Here's how the part is built. I have some questions about the finished solid (model axes, mm). Round coordinates to 2 decimals unless told otherwise and drop trailing zeros. Write each loop counter-clockwise with the first axis right and the second up, starting at its lowest first coordinate (ties: lowest second). Pieces come first, ordered by that corner, then holes. Notation, with made-up numbers: (-18.75, -8) - (39.25, -8) arc R26 cw to (39.25, 18) - close; hole circle Ø2 at (86.5, 60). An arc over 180 degrees is marked (long way). Write item = value, one per line. Start each with the question number.
Item 1: If we section it at C-C (x = 10): Please give me the cut outline in (y, z).
Item 2: If we section it at D-D (y = 0.55): Please give me the cut outline in (x, z).
Item 3: For P1, Ø4.5, axis at x = 35, z = -45, coming from the -Y side, with a flat end and sliding along its axis, tell me the tip position at first contact or that it passes through.
Item 4: If we section it at B-B (z = -10): Please give me the cut outline in (x, y).
Item 5: If we section it at A-A (z = -45): Please give me the cut outline in (x, y).
Item 6: If I drill on line 1 along X through (y, z) = (2.2, -45); line 2 along Z through (x, y) = (36, 2.5); line 3 along X through (y, z) = (0.65, -46), over which ranges is the centre line in solid material (lowest first)? Write a range as [from, to].
```python
from build123d import *

# Parameters (mm, degrees)
SKETCH1_W           = 50
SKETCH1_H           = 50
BOSS_EXTRUDE1_DEPTH = 3
SKETCH2_R           = 2.0066
CUT_EXTRUDE1_DEPTH  = 4
CUT_EXTRUDE2_REACH  = 5
SKETCH3_R           = 1.45


with BuildPart() as part:
    # Sketch1 → Boss-Extrude1 (new body)
    with BuildSketch(Plane(origin=(0, 0, 0), x_dir=(1, 0, 0), z_dir=(0, 1, 0))):
        with Locations((25, 25)):
            Rectangle(SKETCH1_W, SKETCH1_H)
    extrude(amount=BOSS_EXTRUDE1_DEPTH)

    # Sketch2 → Cut-Extrude1 (cut, through all)
    with BuildSketch(Plane(origin=(0, 3, 0), x_dir=(1, 0, 0), z_dir=(0, 1, 0))):
        with Locations((10, 45)):
            Circle(SKETCH2_R)
        with Locations((35, 45)):
            Circle(SKETCH2_R)
        with Locations((10, 10)):
            Circle(SKETCH2_R)
    extrude(amount=-CUT_EXTRUDE1_DEPTH, mode=Mode.SUBTRACT)

    # Sketch3 → Cut-Extrude2 (cut, up to next)
    with BuildSketch(Plane(origin=(0, 3, 0), x_dir=(1, 0, 0), z_dir=(0, 1, 0)), mode=Mode.PRIVATE) as cut_extrude2_sk1:
        with Locations((47.301711452, 25.073921106)):
            Circle(SKETCH3_R)
    cut_extrude2_tool1 = extrude(cut_extrude2_sk1.sketch, amount=-CUT_EXTRUDE2_REACH, mode=Mode.PRIVATE) & part.part
    add(cut_extrude2_tool1.solids().sort_by_distance((47.301711, 3, -25.073921))[0], mode=Mode.SUBTRACT)
    # Sketch3 → Cut-Extrude2 (cut, up to next)
    with BuildSketch(Plane(origin=(0, 3, 0), x_dir=(1, 0, 0), z_dir=(0, 1, 0)), mode=Mode.PRIVATE) as cut_extrude2_sk2:
        with Locations((37.001711452, 2.873921106)):
            Circle(SKETCH3_R)
    cut_extrude2_tool2 = extrude(cut_extrude2_sk2.sketch, amount=-CUT_EXTRUDE2_REACH, mode=Mode.PRIVATE) & part.part
    add(cut_extrude2_tool2.solids().sort_by_distance((37.001711, 3, -2.873921))[0], mode=Mode.SUBTRACT)


solid = part.part
```
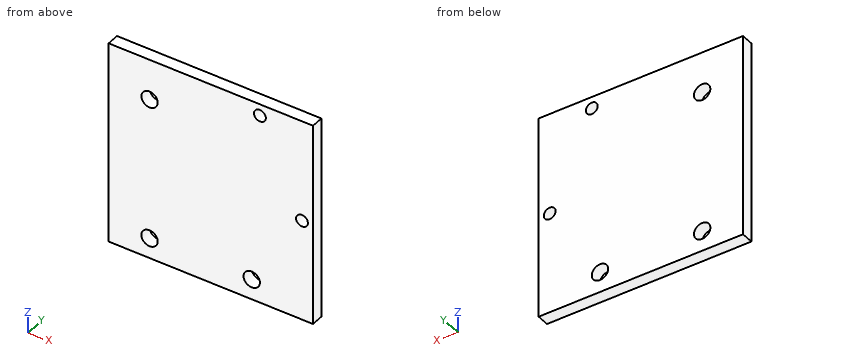
Reply:
q1.outline = (0, -50) - (3, -50) - (3, -47.01) - (0, -47.01) - close; (0, -42.99) - (3, -42.99) - (3, -12.01) - (0, -12.01) - close; (0, -7.99) - (3, -7.99) - (3, 0) - (0, 0) - close
q2.outline = (0, -50) - (50, -50) - (50, 0) - (0, 0) - close; hole circle Ø4.01 at (10, -45); hole circle Ø4.01 at (10, -10); hole circle Ø4.01 at (35, -45); hole circle Ø2.9 at (37, -2.87); hole circle Ø2.9 at (47.3, -25.07)
q3.P1 = 0
q4.outline = (0, 0) - (7.99, 0) - (7.99, 3) - (0, 3) - close; (12.01, 0) - (50, 0) - (50, 3) - (12.01, 3) - close
q5.outline = (0, 0) - (7.99, 0) - (7.99, 3) - (0, 3) - close; (12.01, 0) - (32.99, 0) - (32.99, 3) - (12.01, 3) - close; (37.01, 0) - (50, 0) - (50, 3) - (37.01, 3) - close
q6.line_1 = [0, 7.99], [12.01, 32.99], [37.01, 50]
q6.line_2 = [-50, -46.74], [-43.26, -3.92], [-1.83, 0]
q6.line_3 = [0, 8.26], [11.74, 33.26], [36.74, 50]
